```python
from build123d import *

# Parameters (mm, degrees)
SKETCH_1_R               = 25
EXTRUDE_1_DEPTH          = 2
SKETCH_2_R               = 1.6
CUT_EXTRUDE_1_DEPTH      = 2
PATTERN_CIRCULAR_1_COUNT = 8


with BuildPart() as part:
    # ｽｹｯﾁ1 → ﾎﾞｽ - 押し出し1 (new body)
    with BuildSketch(Plane.XY):
        Circle(SKETCH_1_R)
    extrude(amount=EXTRUDE_1_DEPTH)

    # ｽｹｯﾁ2 → ｶｯﾄ - 押し出し1 (cut)
    with BuildSketch(Plane.XY.offset(2)):
        with Locations((0, 20)):
            Circle(SKETCH_2_R)
        with Locations((-5, 20)):
            Circle(SKETCH_2_R)
    cut_extrude_1 = extrude(amount=-CUT_EXTRUDE_1_DEPTH, mode=Mode.SUBTRACT)

    # 円形ﾊﾟﾀｰﾝ1: ｶｯﾄ - 押し出し1 ×8 about axis
    pattern_circular_1_axis = Axis((0.020649158, -0.165193263, 0), (0, 0, 1))
    for i in range(1, PATTERN_CIRCULAR_1_COUNT):
        add(cut_extrude_1.rotate(pattern_circular_1_axis, i * 360 / PATTERN_CIRCULAR_1_COUNT), mode=Mode.SUBTRACT)


solid = part.part
```
Source: CAD feature listing. Evaluate the final solid. Frame: model axes, mm. Coordinates: 2 decimals unless noted, no trailing zeros. Write each loop counter-clockwise with the first axis right and the second up, starting at its lowest first coordinate (ties: lowest second). Pieces come first, ordered by that corner, then holes. Notation, with made-up numbers: (65, -26.5) -> (108, -26.5) arc R17 ccw to (108, 2.5) -> close; hole circle Ø10 at (-5.75, 38). An arc over 180 degrees is marked (long way). Return JSON: item names as keys, results as strings. Group by question number.
1) Section query D-D, the plane z = 1.45. State how many separate pieces and enclosed holes the cut face has, plus the area to 3 significant figures.
2) Section query C-C, the plane y = -6. Return loops of the section in (x, z).
3) Section query B-B, the plane x = 0. Return loops of the section in (y, z).
4) Section query A-A, the plane y = 20. Return loops of the section in (x, z), plus the area to 3 significant figures.
5) Mould query, pull axis X, two halves, no side actions, for faces 1 (the face through (-13.514, 15.498, 1.014)), 2 (the face through (23.846, 7.509, 0.986)), 3 (the face through (0, 0, 2)). Classes: +X half, -X half, draft (parallel to the pull), parting line (faces both ways), or undercut.
6) Ray query, line 1 along Y through (x, z) = (0, 1.25); line 2 along Y through (x, z) = (-19, 1.2); line 3 along Y through (x, z) = (-13.5, 0.9). Return the intervals inside material, ascending.
From the geometry:
{
 "1": {"separate pieces": "1", "enclosed holes": "16", "area": "1,830 mm²"},
 "2": {"outline": "(-24.27, 0) -> (-21.52, 0) -> (-21.52, 2) -> (-24.27, 2) -> close; (-18.77, 0) -> (24.27, 0) -> (24.27, 2) -> (-18.77, 2) -> close"},
 "3": {"outline": "(-25, 0) -> (-21.93, 0) -> (-21.93, 2) -> (-25, 2) -> close; (-18.73, 0) -> (18.4, 0) -> (18.4, 2) -> (-18.73, 2) -> close; (21.6, 0) -> (25, 0) -> (25, 2) -> (21.6, 2) -> close"},
 "4": {"outline": "(-15, 0) -> (-6.6, 0) -> (-6.6, 2) -> (-15, 2) -> close; (-3.4, 0) -> (-1.6, 0) -> (-1.6, 2) -> (-3.4, 2) -> close; (1.6, 0) -> (15, 0) -> (15, 2) -> (1.6, 2) -> close", "area": "47.2 mm²"},
 "5": {"face 1": "undercut", "face 2": "parting line", "face 3": "draft"},
 "6": {"line 1": "-25 to -21.93, -18.73 to 18.4, 21.6 to 25", "line 2": "-16.25 to -6.3, -4.07 to -1.3, 0.93 to 9.5, 11.59 to 16.25", "line 3": "-21.04 to -15.87, -13.01 to 12.67, 15.49 to 21.04"}
}
